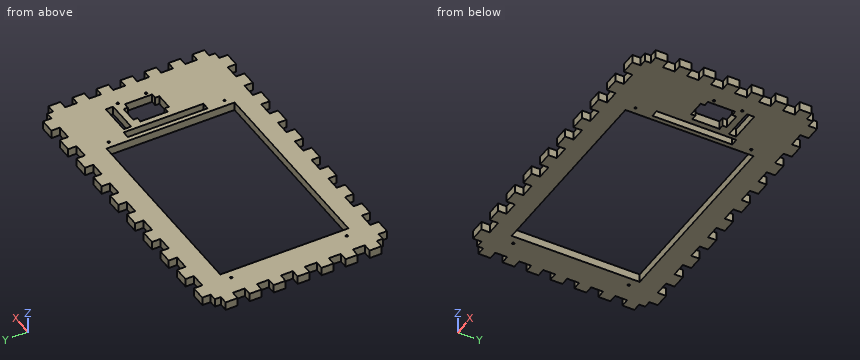
```python
from build123d import *

# Parameters (mm, degrees)
SCHIZZO1_W                   = 140
SCHIZZO1_H                   = 80
SCHIZZO1_R                   = 0.5
SCHIZZO1_W_2                 = 95
SCHIZZO1_H_2                 = 61
SCHIZZO1_W_3                 = 3.5
SCHIZZO1_H_3                 = 38
SCHIZZO1_W_4                 = 15
SCHIZZO1_H_4                 = 3.5
ESTRUSIONE_ESTRUSIONE1_DEPTH = 4
SCHIZZO2_W                   = 7
SCHIZZO2_H                   = 4
ESTRUSIONE_ESTRUSIONE2_DEPTH = 4
RIPETIZIONE_A_L1_COUNT       = 10
RIPETIZIONE_A_L1_PITCH       = 14
SCHIZZO3_W                   = 4
SCHIZZO3_H                   = 5.714285714
ESTRUSIONE_ESTRUSIONE3_DEPTH = 4
RIPETIZIONE_A_L2_COUNT       = 7
RIPETIZIONE_A_L2_PITCH       = 11.428571429


with BuildPart() as part:
    # Schizzo1 → Estrusione-Estrusione1 (new body)
    with BuildSketch(Plane.XY):
        with Locations((70, 40)):
            Rectangle(SCHIZZO1_W, SCHIZZO1_H)
        with Locations((9, 12)):
            Circle(SCHIZZO1_R, mode=Mode.SUBTRACT)
        with Locations((60.5, 39.5)):
            Rectangle(SCHIZZO1_W_2, SCHIZZO1_H_2, mode=Mode.SUBTRACT)
        with Locations((111.2, 12)):
            Circle(SCHIZZO1_R, mode=Mode.SUBTRACT)
        with Locations((111.95, 39.6)):
            Rectangle(SCHIZZO1_W_3, SCHIZZO1_H_3, mode=Mode.SUBTRACT)
        with Locations((131.4, 37.8)):
            Circle(SCHIZZO1_R, mode=Mode.SUBTRACT)
        with Locations((9, 67.1)):
            Circle(SCHIZZO1_R, mode=Mode.SUBTRACT)
        Polygon((119, 36), (116.5, 36), (116.5, 49), (119, 49), (119, 51), (127, 51), (127, 49), (129.5, 49), (129.5, 36), (127, 36), (127, 34), (119, 34), align=None, mode=Mode.SUBTRACT)
        with Locations((131.4, 51.3)):
            Circle(SCHIZZO1_R, mode=Mode.SUBTRACT)
        with Locations((123, 55.75)):
            Rectangle(SCHIZZO1_W_4, SCHIZZO1_H_4, mode=Mode.SUBTRACT)
        with Locations((111.2, 67.1)):
            Circle(SCHIZZO1_R, mode=Mode.SUBTRACT)
    extrude(amount=ESTRUSIONE_ESTRUSIONE1_DEPTH)

    # Schizzo2 → Estrusione-Estrusione2 (add)
    with BuildSketch(Plane.XY.offset(4)):
        with Locations((7, 82)):
            Rectangle(SCHIZZO2_W, SCHIZZO2_H)
        with Locations((7, -2)):
            Rectangle(SCHIZZO2_W, SCHIZZO2_H)
    estrusione_estrusione2 = extrude(amount=-ESTRUSIONE_ESTRUSIONE2_DEPTH)

    # Ripetizione a L1: Estrusione-Estrusione2 ×10
    with Locations(*[(i * RIPETIZIONE_A_L1_PITCH, 0, 0) for i in range(1, RIPETIZIONE_A_L1_COUNT)]):
        add(estrusione_estrusione2)

    # Schizzo3 → Estrusione-Estrusione3 (add)
    with BuildSketch(Plane.XY.offset(4)):
        with Locations((-2, 74.285714286)):
            Rectangle(SCHIZZO3_W, SCHIZZO3_H)
        with Locations((142, 74.285714286)):
            Rectangle(SCHIZZO3_W, SCHIZZO3_H)
    estrusione_estrusione3 = extrude(amount=-ESTRUSIONE_ESTRUSIONE3_DEPTH)

    # Ripetizione a L2: Estrusione-Estrusione3 ×7
    with Locations(*[(0, -i * RIPETIZIONE_A_L2_PITCH, 0) for i in range(1, RIPETIZIONE_A_L2_COUNT)]):
        add(estrusione_estrusione3)


solid = part.part
```
Source: CAD feature listing. Evaluate the final solid. Frame: model axes, mm. Coordinates: 2 decimals unless noted, no trailing zeros. Loops run counter-clockwise (first coordinate to the right, second up) from the corner with the lowest first, then second, coordinate; pieces in that order, holes last. Notation, with made-up numbers: M 83,-13 L 90,-13 A15 cw 90,0 Z; hole C 78,-27.75 d11. An arc over 180 degrees is marked long. Put each result on its own line as item: value. Start each with the question number.
1) Cut plane B-B on z = 3.4. Give the number of separate pieces and of enclosed holes in the cut face, then the cut area to 3 significant figures.
2) Ray query, L1, parallel to X at y = 22, z = 2.25; L2, parallel to X at y = 43.5, z = 2.6; L3, parallel to Y at x = 111.2, z = 2.1. Return the intervals inside material, ascending. Write a range as from..to.
3) Cut plane A-A on x = 120.5. Return the cut outline in (y, z), then the cut area to 3 significant figures.
4) Contact query for flat-ended pins moving along their axis: pin 1 Ø1 at (y, z) = (35.5, 1) entering from -X; pin 2 Ø1.2 at (x, z) = (43, 3) entering from -Y; pin 3 Ø1.2 at (y, z) = (-1.5, 1.5) entering from -X. Output: stop coordinate, or through.
The answers:
1. separate pieces: 1
1. enclosed holes: 10
1. area: 5,890 mm²
2. L1: x = 0..13, 108..110.2, 113.7..140
2. L2: x = 0..13, 108..110.2, 113.7..116.5, 129.5..140
2. L3: y = 0..11.5, 12.5..20.6, 58.6..66.6, 67.6..80
3. outline: M -4,0 L 34,0 L 34,4 L -4,4 Z; M 51,0 L 54,0 L 54,4 L 51,4 Z; M 57.5,0 L 84,0 L 84,4 L 57.5,4 Z
3. area: 270 mm²
4. pin 1: stops at x = 0
4. pin 2: stops at y = 0
4. pin 3: stops at x = 3.5
